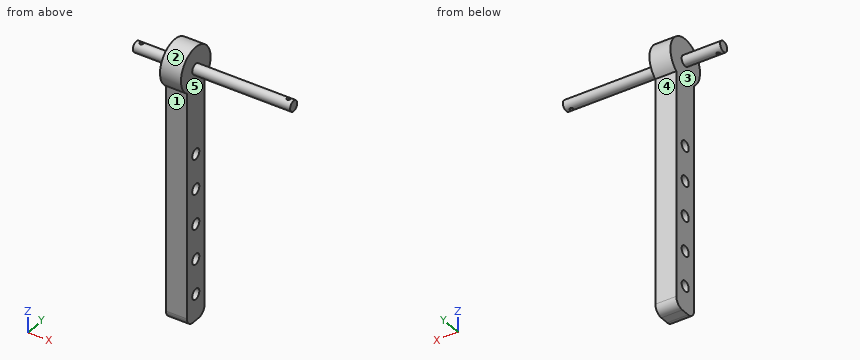
from build123d import *

# Parameters (mm, degrees)
SKETCH_1_W           = 150
SKETCH_1_H           = 15
EXTRUDE_1_DEPTH      = 12
FILLET_1_R           = 5
SKETCH_6_R           = 12.5
EXTRUDE_2_DEPTH      = 12
EXTRUDE_5_DEPTH      = 22
EXTRUDE_5_DEPTH_BACK = 68
SKETCH_15_R          = 3
CUT_EXTRUDE_9_REACH  = 167.904
SKETCH_16_R          = 1
CUT_EXTRUDE_10_REACH = 167.904
SKETCH_17_R          = 3


with BuildPart() as part:
    # 草图1 → 凸台-拉伸1 (new body)
    with BuildSketch(Plane(origin=(0, 0, 0), x_dir=(0, 0, -1), z_dir=(1, 0, 0))):
        with Locations((75, 7.5)):
            Rectangle(SKETCH_1_W, SKETCH_1_H)
    extrude(amount=EXTRUDE_1_DEPTH)

    # 圆角1
    fillet_1_edges = [part.edges().sort_by_distance(p)[0] for p in [
        (6, 15, 0),
        (6, 15, -150),
        (6, 0, -150),
        (6, 0, 0),
    ]]
    fillet(fillet_1_edges, radius=FILLET_1_R)

    # 草图6 → 凸台-拉伸2 (add)
    with BuildSketch(Plane(origin=(12, 0, 0), x_dir=(0, 0, -1), z_dir=(1, 0, 0))):
        with Locations((6.4, 7.5)):
            Circle(SKETCH_6_R)
    extrude(amount=-EXTRUDE_2_DEPTH)

    # 草图15 → 凸台-拉伸5 (add, two sides: drawn at the far end of the back side and taken through both)
    with BuildSketch(Plane.ZY.offset(-EXTRUDE_5_DEPTH_BACK)):
        with Locations((-6.4, 7.5)):
            Circle(SKETCH_15_R)
    extrude(amount=EXTRUDE_5_DEPTH + EXTRUDE_5_DEPTH_BACK)

    # 草图16 → 切除-拉伸9 (cut, up to next)
    with BuildSketch(Plane.XY, mode=Mode.PRIVATE) as cut_extrude_9_sk1:
        with Locations((-19, 7.5)):
            Circle(SKETCH_16_R)
    cut_extrude_9_tool1 = extrude(cut_extrude_9_sk1.sketch, amount=-CUT_EXTRUDE_9_REACH, mode=Mode.PRIVATE) & part.part
    # 草图16 → 切除-拉伸9 (cut, up to next)
    with BuildSketch(Plane.XY, mode=Mode.PRIVATE) as cut_extrude_9_sk2:
        with Locations((65, 7.5)):
            Circle(SKETCH_16_R)
    cut_extrude_9_tool2 = extrude(cut_extrude_9_sk2.sketch, amount=-CUT_EXTRUDE_9_REACH, mode=Mode.PRIVATE) & part.part
    add(cut_extrude_9_tool1.solids().sort_by_distance((-19, 7.5, 0))[0], mode=Mode.SUBTRACT)
    add(cut_extrude_9_tool2.solids().sort_by_distance((65, 7.5, 0))[0], mode=Mode.SUBTRACT)

    # 草图17 → 切除-拉伸10 (cut, up to next)
    with BuildSketch(Plane.ZY, mode=Mode.PRIVATE) as cut_extrude_10_sk1:
        with Locations((-135, 7.5)):
            Circle(SKETCH_17_R)
    cut_extrude_10_tool1 = extrude(cut_extrude_10_sk1.sketch, amount=-CUT_EXTRUDE_10_REACH, mode=Mode.PRIVATE) & part.part
    # 草图17 → 切除-拉伸10 (cut, up to next)
    with BuildSketch(Plane.ZY, mode=Mode.PRIVATE) as cut_extrude_10_sk2:
        with Locations((-115, 7.5)):
            Circle(SKETCH_17_R)
    cut_extrude_10_tool2 = extrude(cut_extrude_10_sk2.sketch, amount=-CUT_EXTRUDE_10_REACH, mode=Mode.PRIVATE) & part.part
    # 草图17 → 切除-拉伸10 (cut, up to next)
    with BuildSketch(Plane.ZY, mode=Mode.PRIVATE) as cut_extrude_10_sk3:
        with Locations((-95, 7.5)):
            Circle(SKETCH_17_R)
    cut_extrude_10_tool3 = extrude(cut_extrude_10_sk3.sketch, amount=-CUT_EXTRUDE_10_REACH, mode=Mode.PRIVATE) & part.part
    # 草图17 → 切除-拉伸10 (cut, up to next)
    with BuildSketch(Plane.ZY, mode=Mode.PRIVATE) as cut_extrude_10_sk4:
        with Locations((-75, 7.5)):
            Circle(SKETCH_17_R)
    cut_extrude_10_tool4 = extrude(cut_extrude_10_sk4.sketch, amount=-CUT_EXTRUDE_10_REACH, mode=Mode.PRIVATE) & part.part
    # 草图17 → 切除-拉伸10 (cut, up to next)
    with BuildSketch(Plane.ZY, mode=Mode.PRIVATE) as cut_extrude_10_sk5:
        with Locations((-55, 7.5)):
            Circle(SKETCH_17_R)
    cut_extrude_10_tool5 = extrude(cut_extrude_10_sk5.sketch, amount=-CUT_EXTRUDE_10_REACH, mode=Mode.PRIVATE) & part.part
    add(cut_extrude_10_tool1.solids().sort_by_distance((0, 7.5, -135))[0], mode=Mode.SUBTRACT)
    add(cut_extrude_10_tool2.solids().sort_by_distance((0, 7.5, -115))[0], mode=Mode.SUBTRACT)
    add(cut_extrude_10_tool3.solids().sort_by_distance((0, 7.5, -95))[0], mode=Mode.SUBTRACT)
    add(cut_extrude_10_tool4.solids().sort_by_distance((0, 7.5, -75))[0], mode=Mode.SUBTRACT)
    add(cut_extrude_10_tool5.solids().sort_by_distance((0, 7.5, -55))[0], mode=Mode.SUBTRACT)


solid = part.part
Can you work these out from the model? Positions are in its coordinate system, mm. Face numbers are marked on the shaded views. A direction names the side the tool comes from. Give positions to 0.01 mm unless a question says otherwise; leave off trailing zeros. Loops run counter-clockwise (first coordinate to the right, second up) from the corner with the lowest first, then second, coordinate; pieces in that order, holes last. Notation, with made-up numbers: (87.25, 9.25) -> (108.25, 9.25) arc R19 ccw to (108.25, 13.25) -> close; hole circle Ø1 at (19.25, -24). An arc over 180 degrees is marked (long way). Write item = value, one per line.
1) Will these pins go through, and if not, where does the flat tip stop? pin 1 (5 mm diameter, centred on y = 7.5, z = -75, fed in from -X); pin 2 (5 mm diameter, centred on y = 6, z = -103, fed in from +X); pin 3 (2.5 mm diameter, centred on x = -19, y = 7.5, fed in from +Z); pin 4 (2 mm diameter, centred on x = 7.5, z = -15.5, fed in from -Y).
Check result:
pin_1 = through
pin_2 = 12
pin_3 = -3.4
pin_4 = -2.02
2) Suppose I cut it at C-C on x = 20. Write out the boundary of the cut face in (y, z), then the cut area to 3 significant figures.
Check result:
outline = circle Ø6 at (7.5, -6.4)
area = 28.3 mm2
3) Suppose I cut it at A-A on z = -6.4. Write out the boundary of the cut face in (x, y), then the cut area to 3 significant figures.
Check result:
outline = (-22, 4.5) -> (0, 4.5) -> (0, -5) -> (12, -5) -> (12, 4.5) -> (68, 4.5) -> (68, 10.5) -> (12, 10.5) -> (12, 20) -> (0, 20) -> (0, 10.5) -> (-22, 10.5) -> close; hole circle Ø2 at (-19, 7.5); hole circle Ø2 at (65, 7.5)
area = 762 mm2
4) I need wall thicknesses on L1, parallel to X at y = 7.5, z = -4.5; L2, parallel to Y at x = 9, z = -75; L3, parallel to X at y = 7.75, z = -44.5. Which ranges of each line are inside material? Lowest first, please. Write a range as from..to.
Check result:
L1 = -22..-20, -18..64, 66..68
L2 = 0..4.5, 10.5..15
L3 = 0..12
5) Suppose I cut it at B-B on z = -95. Write out the boundary of the cut face in (x, y).
Check result:
outline = (0, 0) -> (12, 0) -> (12, 4.5) -> (0, 4.5) -> close; (0, 10.5) -> (12, 10.5) -> (12, 15) -> (0, 15) -> close
6) Thinking about a two-plate mould opening in X: for the marked faces 3, 4 and 5, which applies, released by +X, released by -X, zero draft, split by the parting line, or undercut?
Check result:
face_3 = released by -X
face_4 = zero draft
face_5 = released by +X
7) For the marked faces 1 and 2, which set-ups out of +Z, -Z, +X, -X, +Y, -Y let a thin tool reach every point of the face, with its end or its side?
Check result:
face_1 = -Z, +X, -X, -Y
face_2 = +X, -X
8) Suppose I cut it at D-D on y = -3. Write out the boundary of the cut face in (x, z).
Check result:
outline = (0, -13.18) -> (12, -13.18) -> (12, 0.38) -> (0, 0.38) -> close
